Check sheet for the modelled part. Datum: model origin and axes. Units: mm. Coordinates: 2 decimals unless noted, no trailing zeros. Write each loop counter-clockwise with the first axis right and the second up, starting at its lowest first coordinate (ties: lowest second). Pieces come first, ordered by that corner, then holes. Notation, with made-up numbers: M 49,14 L 78,14 A16 cw 78,41 Z; hole C 16,-32 d10. An arc over 180 degrees is marked long. Answer as CSV lines item,"result". Start each with the question number.
Q1. Sectioned sample at B-B, the plane x = 4.25. Record the cut outline in (y, z), then the cut area to 3 significant figures.
Q2. Sectioned sample at C-C, the plane z = 5. Record the cut outline in (x, y).
Q3. Depth check by flat-ended pin: pin 1 Ø2 at (y, z) = (2, -15.5) entering from -X; pin 2 Ø5 at (y, z) = (-3.5, 12.5) entering from -X; pin 3 Ø5 at (y, z) = (-5.5, -8) entering from +X. Enter the tip coordinate at first touch or a pass-through.
Q4. Thickness scan on line 1 along Y through (x, z) = (2, -5); line 2 along X through (y, z) = (1, 14); line 3 along X through (y, z) = (6.75, 1). Record the ranges inside material, lowest first. Write a range as from..to.
Q5. Sectioned sample at A-A, the plane y = -3. Record the cut outline in (x, z), then the cut area to 3 significant figures.
Q6. Sectioned sample at D-D, the plane z = -16.5. Record the cut outline in (x, y), then the cut area to 3 significant figures.
from build123d import *

# Parameters (mm, degrees)
F3_DEPTH = 12.7
F4_DEPTH = 12.7
F5_ANGLE = 90


with BuildPart() as f3:
    # F0 (on Front) → F3 (new body, symmetric)
    with BuildSketch(Plane.XZ):
        Polygon((7.784226, 0), (0, 18.228879), (-7.784226, 0), (0, -30.053018), align=None)
    extrude(amount=F3_DEPTH, both=True)


with BuildPart() as f4:
    # F1 (on Front) → F4 (new body, symmetric)
    with BuildSketch(Plane.XZ):
        Polygon((-7.784226, 0), (0, -30.053018), (7.784226, 0), (0, 18.228879), align=None)
    extrude(amount=F4_DEPTH, both=True)


with BuildPart() as f3_1:
    # F5: moved
    add(f3.part.rotate(Axis((0, 0, -12.11974), (0, 0, -1)), F5_ANGLE))


with BuildPart() as f4_1:
    add(f4.part)

    # F6: intersect F3
    add(f3_1.part, mode=Mode.INTERSECT)


solid = f4_1.part
Output:
1,outline,"M -7.78,0 L -4.25,-13.64 L 4.25,-13.64 L 7.78,0 L 4.25,8.28 L -4.25,8.28 Z"
1,area,"264 mm^2"
2,outline,"M -5.65,-5.65 L 5.65,-5.65 L 5.65,5.65 L -5.65,5.65 Z"
3,pin 1,"stops at x = -4.03"
3,pin 2,"stops at x = -3.51"
3,pin 3,"stops at x = 6.36"
4,line 1,"y = -6.49..6.49"
4,line 2,"x = -1.81..1.81"
4,line 3,"x = -7.36..7.36"
5,outline,"M -7.78,0 L -3,-18.47 L 3,-18.47 L 7.78,0 L 3,11.2 L -3,11.2 Z"
5,area,"320 mm^2"
6,outline,"M -3.51,-3.51 L 3.51,-3.51 L 3.51,3.51 L -3.51,3.51 Z"
6,area,"49.3 mm^2"
